The model under review builds one solid part; all positions refer to its coordinate system, in mm. A direction names the side the tool comes from. Coordinates: 2 decimals unless noted, no trailing zeros. Loops run counter-clockwise (first coordinate to the right, second up) from the corner with the lowest first, then second, coordinate; pieces in that order, holes last. Notation, with made-up numbers: (68, 70.5) - (102, 70.5) arc R20 cw to (102, 105.5) - close; hole circle Ø10 at (11.5, 2). An arc over 180 degrees is marked (long way). Answer in a Markdown table with one row per item. Add a question column.
(1) For line 1 along Z through (x, y) = (0, -2.3); line 2 along Y through (x, z) = (-12.5, 20.3); line 3 along Z through (x, y) = (25, 7), list the stretches that pass through material, from the lowest coordinate up.
(2) We need section D-D on y = -2. Write out the cut boundary in (x, z), plus the area to 3 significant figures.
(3) We need section A-A on x = 25. Write out the cut boundary in (y, z), plus the area to 3 significant figures.
(4) Mouldability with a two-part tool opening along Z and no side actions: class faces 1 (the cylindrical face through (22.253, 5.112, -0.121)), 2 (the flat face through (13, 2, 25)), 3 (the flat face through (13, 10, 13)) as +Z half, -Z half, draft (parallel to the pull), parting line (faces both ways), or undercut.
(5) Machinability: for faces 4 (the cylindrical face through (21.8, -1.5, 2.4)), 5 (the flat face through (-8.5, 5, 17)), 6 (the flat face through (18.656, 5, 11)), 7 (the cylindrical face through (6.518, 4.93, -4.188)), 8 (the flat face through (6.344, 5, 11)), which of the approach directions +Z, -Z, +X, -X, +Y, -Y give a long, thin tool a straight path to every point of the face, cutting with its end or side? Answer none if there is none.
(6) For P1, Ø6.5, axis at x = -12.5, y = 5, coming from the -Z side; P2, Ø5, axis at y = 7.5, z = 0, coming from the -X side; P3, Ø1, axis at y = 10, z = 12.5, coming from the +X side, all flat-tipped, find the tip position at first contact; note any pin that passes through.
(7) We need section B-B on z = 17. Write out the cut boundary in (x, y).
Autodesk Inventor part; units mm, degrees
ref_plane "YZ Plane" through (0, 0, 0) normal (1, 0, 0) x (0, 1, 0)
ref_plane "XZ Plane" through (0, 0, 0) normal (0, 1, 0) x (-1, 0, 0)
ref_plane "XY Plane" through (0, 0, 0) normal (0, 0, 1) x (1, 0, 0)
sketch "Sketch4" plane through (0, 0, 0) normal (0, 1, 0) x (-1, 0, 0)
  circle A0 centre (0, 0) radius 7.5
  circle A1 centre (0, 0) radius 2.75
  dimension "d19" = 15
  dimension "d20" = 5.5
extrude "Extrusion4" add sketch "Sketch4" along normal blind 10
ref_plane "Work Plane2" through (0, 5, 0) normal (0, 1, 0) x (1, 0, 0)
sketch "Sketch12" plane through (0, 5, 0) normal (0, 1, 0) x (1, 0, 0)
  circle A0 centre (0, 0) radius 2.75
  line L0 (0, 0) -> (25, 0)
  circle A1 centre (25, 0) radius 2.75
  circle A2 centre (25, 0) radius 7.5
  line L1 (12.5, 0) -> (12.5, -20)
  line L2 (42.5, -25) -> (-17.5, -25)
  line L3 (-17.5, -25) -> (-17.5, -15)
  line L4 (-17.5, -15) -> (42.5, -15)
  line L5 (42.5, -15) -> (42.5, -25)
  line L6 (42.5, -25) -> (-17.5, -15) construction
  line L7 (-17.5, -25) -> (42.5, -15) construction
  circle A3 centre (0, 0) radius 7.5
  line L8 (18.6557, -4) -> (6.3443, -4)
  line L9 (6.3443, -4) -> (6.3443, 4)
  line L10 (6.3443, 4) -> (18.6557, 4)
  line L11 (18.6557, 4) -> (18.6557, -4)
  line L12 (18.6557, -4) -> (6.3443, 4) construction
  line L13 (6.3443, -4) -> (18.6557, 4) construction
  line L14 (6.3443, 4) -> (18.6557, 4)
  line L15 (18.6557, 4) -> (18.6557, -16)
  line L16 (18.6557, -16) -> (6.3443, -16)
  line L17 (6.3443, -16) -> (6.3443, 4)
  point P0 (6.3443, -15)
  point P1 (18.6557, -15)
  dimension "d66" = 25
  dimension "d67" = 5.5
  dimension "d68" = 15
  dimension "d69" = 20
  dimension "d70" = 60
  dimension "d71" = 10
  dimension "d72" = 8
  dimension "d73" = 20
extrude "Extrusion10" add sketch "Sketch12" along normal mid plane 10 contours A3 L10 A2 L0 | L0 L1 L8 A3 | L8 L1 L4 L17 | L0 A2 L8 L1 | L8 L15 L4 L1 | L17 L16 L15 L4 L5 L2 L3 | L4 L1 L16 L17 | L11 L0 A2 | A2 L11 | L0 L11 A2 | L4 L15 L16 L1
sketch "Sketch13" plane through (18.6557, 10, -4) normal (0, 0, -1) x (-1, 0, 0)
  line L0 (0, 0) -> (12.3114, 0)
  line L1 (6.1557, 0) -> (6.1557, -5)
  line L2 (6.1557, -9.6188) -> (2.1557, -7.3094)
  line L3 (2.1557, -7.3094) -> (2.1557, -2.6906)
  line L4 (2.1557, -2.6906) -> (6.1557, -0.3812)
  line L5 (6.1557, -0.3812) -> (10.1557, -2.6906)
  line L6 (10.1557, -2.6906) -> (10.1557, -7.3094)
  line L7 (10.1557, -7.3094) -> (6.1557, -9.6188)
  line L8 (36.1557, -10) -> (36.1557, 0)
  line L9 (36.1557, -5) -> (31.1557, -5)
  line L10 (31.1557, -9.6188) -> (27.1557, -7.3094)
  line L11 (27.1557, -7.3094) -> (27.1557, -2.6906)
  line L12 (27.1557, -2.6906) -> (31.1557, -0.3812)
  line L13 (31.1557, -0.3812) -> (35.1557, -2.6906)
  line L14 (35.1557, -2.6906) -> (35.1557, -7.3094)
  line L15 (35.1557, -7.3094) -> (31.1557, -9.6188)
  line L16 (-23.8443, -10) -> (-23.8443, 0)
  line L17 (-23.8443, -5) -> (-18.8443, -5)
  line L18 (-23.8443, -5) -> (-18.8443, -5) construction
  line L19 (-18.8443, -9.6188) -> (-22.8443, -7.3094)
  line L20 (-22.8443, -7.3094) -> (-22.8443, -2.6906)
  line L21 (-22.8443, -2.6906) -> (-18.8443, -0.3812)
  line L22 (-18.8443, -0.3812) -> (-14.8443, -2.6906)
  line L23 (-14.8443, -2.6906) -> (-14.8443, -7.3094)
  line L24 (-14.8443, -7.3094) -> (-18.8443, -9.6188)
  point P0 (18.6557, -10)
  dimension "d76" = 5
  dimension "d77" = 8
  dimension "d78" = 5
  dimension "d79" = 8
  dimension "d80" = 5
  dimension "d81" = 0
  dimension "d82" = 8
extrude "Extrusion11" cut sketch "Sketch13" against normal blind 23
fillet "Fillet4" radius 2 8 edges at (18.6557, 5, 15) (6.3443, 5, 15) (-17.5, 5, 25) (42.5, 5, 25) (6.3443, 5, -4) (18.6557, 5, -4) (18.6557, 5, 4) (6.3443, 5, 4)
sketch "Sketch14" plane through (17.6345, 0, -4) normal (0, 0, -1) x (-1, 0, 0)
  circle A0 centre (5.2691, 5) radius 2.75
  line L0 (0, 10) -> (10.2691, 10)
  line L1 (10.2691, 10) -> (10.2691, 0)
  circle A1 centre (-19.8655, 5) radius 2.75
  circle A2 centre (30.1345, 5) radius 2.75
  line L2 (35.1345, 0) -> (35.1345, 10)
  line L3 (-24.8655, 0) -> (-24.8655, 10)
  point P0 (17.6345, 0)
  dimension "d86" = 5.5
  dimension "d87" = 5
  dimension "d88" = 5
  dimension "d89" = 5.5
  dimension "d90" = 5.5
  dimension "d91" = 5
  dimension "d92" = 5
extrude "Extrusion12" cut sketch "Sketch14" against normal through all
sketch "Sketch15" plane through (0, 10, 0) normal (0, 1, 0) x (1, 0, 0)
  circle A0 centre (0, 0) radius 2.75
  circle A1 centre (25, 0) radius 2.75
  circle A2 centre (25, 0) radius 2.75
  circle A3 centre (0, 0) radius 2.75
  circle A4 centre (0, 0) radius 4
  circle A5 centre (25, 0) radius 4
  dimension "d95" = 5.5
  dimension "d96" = 5.5
  dimension "d97" = 8
  dimension "d98" = 8
extrude "Extrusion13" add sketch "Sketch15" along normal blind 3
sketch "Sketch16" plane through (0, 0, 0) normal (0, -1, 0) x (1, 0, 0)
  circle A0 centre (0, 0) radius 2.75
  circle A1 centre (0, 0) radius 2.75
  circle A2 centre (25, 0) radius 2.75
  circle A3 centre (25, 0) radius 2.75
  circle A4 centre (25, 0) radius 4
  circle A5 centre (0, 0) radius 4
  dimension "d101" = 5.5
  dimension "d102" = 8
  dimension "d103" = 8
extrude "Extrusion14" add sketch "Sketch16" along normal blind 3
properties part number "4mm_Roller_Spacer" material "PET Plastic"
Outcome:
| question | item | result |
|---|---|---|
| 1 | line 1 | -4 to -2.75, 2.75 to 4 |
| 1 | line 2 | 0 to 2.25, 7.75 to 10 |
| 1 | line 3 | -7.5 to -2.75, 2.75 to 7.5, 15 to 25 |
| 2 | outline | circle Ø8 at (0, 0); circle Ø8 at (25, 0); hole circle Ø5.5 at (0, 0); hole circle Ø5.5 at (25, 0) |
| 2 | area | 53.0 mm² |
| 3 | outline | (-3, -4) - (0, -4) - (0, -7.5) - (10, -7.5) - (10, -4) - (13, -4) - (13, -2.75) - (-3, -2.75) - close; (-3, 2.75) - (13, 2.75) - (13, 4) - (10, 4) - (10, 7.5) - (0, 7.5) - (0, 4) - (-3, 4) - close; (0, 15) - (10, 15) - (10, 25) - (0, 25) - close |
| 3 | area | 210 mm² |
| 4 | face 1 | undercut |
| 4 | face 2 | +Z half |
| 4 | face 3 | draft |
| 5 | face 4 | -Y |
| 5 | face 5 | -Z |
| 5 | face 6 | +X, +Y, -Y |
| 5 | face 7 | -Z, +Y, -Y |
| 5 | face 8 | -X, +Y, -Y |
| 6 | P1 | z = 19 |
| 6 | P2 | x = -7.5 |
| 6 | P3 | x = 18.66 |
| 7 | outline | (-17.5, 0) - (42.5, 0) - (42.5, 10) - (-17.5, 10) - close; hole (-16.5, 2.69) - (-12.5, 0.38) - (-8.5, 2.69) - (-8.5, 7.31) - (-12.5, 9.62) - (-16.5, 7.31) - close; hole (8.5, 2.69) - (12.5, 0.38) - (16.5, 2.69) - (16.5, 7.31) - (12.5, 9.62) - (8.5, 7.31) - close; hole (33.5, 2.69) - (37.5, 0.38) - (41.5, 2.69) - (41.5, 7.31) - (37.5, 9.62) - (33.5, 7.31) - close |
